```python
from build123d import *

# Parameters (mm, degrees)
CROQUIS1_R              = 1.75
CROQUIS1_R_2            = 1.5
SALIENTE_EXTRUIR1_DEPTH = 9
REDONDEO1_R             = 1


with BuildPart() as part:
    # Croquis1 → Saliente-Extruir1 (new body)
    with BuildSketch(Plane.XY):
        Polygon((0, 34), (0, 0), (10.5, 0), (10.5, -15), (19.5, -15), (19.5, 0), (40.5, 0), (40.5, -15), (49.5, -15), (49.5, 0), (60, 0), (60, 34), align=None)
        with Locations((6.5, 14.5)):
            Circle(CROQUIS1_R, mode=Mode.SUBTRACT)
        with Locations((6.5, 23.5)):
            Circle(CROQUIS1_R, mode=Mode.SUBTRACT)
        with BuildLine():
            Line((10.5, 24.545268253), (10.5, 29))
            Line((10.5, 29), (15.417424305, 29))
            ThreePointArc((15.417424305, 29), (20, 30), (24.582575695, 29))
            Line((24.582575695, 29), (51.5, 29))
            Line((51.5, 29), (51.5, 9))
            Line((51.5, 9), (24.582575695, 9))
            ThreePointArc((24.582575695, 9), (20, 8), (15.417424305, 9))
            Line((15.417424305, 9), (10.5, 9))
            Line((10.5, 9), (10.5, 13.454731747))
            ThreePointArc((10.5, 13.454731747), (9, 19), (10.5, 24.545268253))
        make_face(mode=Mode.SUBTRACT)
        with Locations((55.5, 14.5)):
            Circle(CROQUIS1_R, mode=Mode.SUBTRACT)
        with Locations((55.5, 23.5)):
            Circle(CROQUIS1_R, mode=Mode.SUBTRACT)
        with Locations((15, -7.5)):
            Circle(CROQUIS1_R_2, mode=Mode.SUBTRACT)
        with Locations((45, -7.5)):
            Circle(CROQUIS1_R_2, mode=Mode.SUBTRACT)
    extrude(amount=SALIENTE_EXTRUIR1_DEPTH)

    # Redondeo1
    redondeo1_edges = [part.edges().sort_by_distance(p)[0] for p in [
        (45, -15, 0),
        (15, -15, 0),
        (49.5, -15, 4.5),
        (40.5, -15, 4.5),
        (19.5, -15, 4.5),
        (10.5, -15, 4.5),
        (15, -15, 9),
        (45, -15, 9),
    ]]
    fillet(redondeo1_edges, radius=REDONDEO1_R)


solid = part.part
```
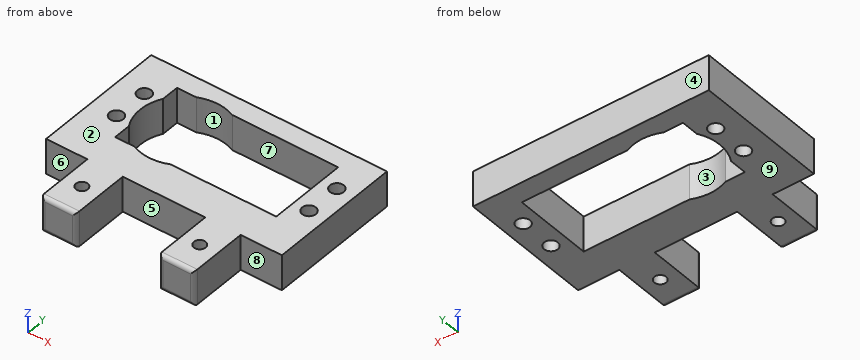
Read the model definition and answer for the solid it produces. Units are mm, in the model's axes. Face numbers are marked on the shaded views. A direction names the side the tool comes from. Round coordinates to 2 decimals unless told otherwise and drop trailing zeros. Write each loop counter-clockwise with the first axis right and the second up, starting at its lowest first coordinate (ties: lowest second). Pieces come first, ordered by that corner, then holes. Notation, with made-up numbers: (-17.75, 12.25) -> (26.25, 12.25) arc R13 cw to (26.25, 26.25) -> close; hole circle Ø6 at (46, 9.25). An arc over 180 degrees is marked (long way). Answer in a Markdown table with one row per item. Add a question column.
1) Determine the mould class of the marked faces 1, 2, 3 and 4 for opening direction Y: pulls with the +Y half, pulls with the -Y half, needs draft (parallel to the pull), parting line crosses it, or undercut.
2) Which of the six approach directions +Z, -Z, +X, -X, +Y, -Y give full straight-line access (tool end or side, diameter ignored) to the marked faces 5, 6, 7, 8 and 9?
3) Find section C-C, the plane z = 5.25. State how many separate pieces and enclosed holes the cut face has, and give its area (3 significant figures).
4) Find section D-D, the plane x = 38.5. Determine the outline of the cut face in (y, z).
5) Find section A-A, the plane x = 45. Determine the outline of the cut face in (y, z), and give its area (3 significant figures).
6) Given P1, Ø4.5, axis at y = -7, z = 3.5, coming from the +X side; P2, Ø4, axis at y = -2.5, z = 5, coming from the -X side, each flat-ended and moving along its own axis, determine where each tip first touches the part or whether it passes through.
7) Consider line 1 (Y direction, x = 6.5, z = 7); line 2 (Y direction, x = 15, z = 2.25); line 3 (X direction, y = -8, z = 0.5). Determine where each line is inside the solid, lowest interval first.
8) Find section B-B, the plane y = 27.5. Determine the outline of the cut face in (x, z).
Findings below:
| question | item | result |
|---|---|---|
| 1 | face 1 | undercut |
| 1 | face 2 | needs draft |
| 1 | face 3 | undercut |
| 1 | face 4 | pulls with the +Y half |
| 2 | face 5 | +Z, -Z, -Y |
| 2 | face 6 | +Z, -Z, -X, -Y |
| 2 | face 7 | +Z, -Z |
| 2 | face 8 | +Z, -Z, +X, -Y |
| 2 | face 9 | -Z, +X, -X, +Y, -Y |
| 3 | separate pieces | 1 |
| 3 | enclosed holes | 7 |
| 3 | area | 1,410 mm² |
| 4 | outline | (0, 0) -> (9, 0) -> (9, 9) -> (0, 9) -> close; (29, 0) -> (34, 0) -> (34, 9) -> (29, 9) -> close |
| 5 | outline | (-15, 1) arc R1 ccw to (-14, 0) -> (-9, 0) -> (-9, 9) -> (-14, 9) arc R1 ccw to (-15, 8) -> close; (-6, 0) -> (9, 0) -> (9, 9) -> (-6, 9) -> close; (29, 0) -> (34, 0) -> (34, 9) -> (29, 9) -> close |
| 5 | area | 234 mm² |
| 6 | P1 | x = 49.5 |
| 6 | P2 | x = 10.5 |
| 7 | line 1 | 0 to 12.75, 16.25 to 21.75, 25.25 to 34 |
| 7 | line 2 | -15 to -9, -6 to 9, 29 to 34 |
| 7 | line 3 | 10.5 to 13.59, 16.41 to 19.5, 40.5 to 43.59, 46.41 to 49.5 |
| 8 | outline | (0, 0) -> (10.5, 0) -> (10.5, 9) -> (0, 9) -> close; (51.5, 0) -> (60, 0) -> (60, 9) -> (51.5, 9) -> close |
